Work out the finished part from the listing and answer in its coordinate system (mm). A direction names the side the tool comes from. Give positions to 0.01 mm unless a question says otherwise; leave off trailing zeros. Loops run counter-clockwise (first coordinate to the right, second up) from the corner with the lowest first, then second, coordinate; pieces in that order, holes last.
from build123d import *

# Parameters (mm, degrees)
SKETCH1_W           = 325
SKETCH1_H           = 10
SKETCH1_W_2         = 10
SKETCH1_H_2         = 34.925125471
BOSS_EXTRUDE1_DEPTH = 190
SKETCH2_W           = 190
SKETCH2_H           = 7.5
BOSS_EXTRUDE2_DEPTH = 5
SKETCH6_W           = 43.6
SKETCH6_H           = 10
BOSS_EXTRUDE4_DEPTH = 190
CUT_EXTRUDE1_START  = -45.92512547
SKETCH3_W           = 153.75
SKETCH3_H           = 43.596922071
CUT_EXTRUDE1_DEPTH  = 56.92512547
SKETCH4_R           = 2.5
BOSS_EXTRUDE3_DEPTH = 171.875
LPATTERN1_COUNT     = 2
LPATTERN1_PITCH     = 190
SKETCH7_W           = 176
SKETCH7_H           = 27.925125471
CUT_EXTRUDE5_DEPTH  = 315
SKETCH8_W           = 25
SKETCH8_H           = 10
BOSS_EXTRUDE6_DEPTH = 325


with BuildPart() as part:
    # Sketch1 → Boss-Extrude1 (new body)
    with BuildSketch(Plane(origin=(0, 0, 0), x_dir=(0, 0, -1), z_dir=(1, 0, 0))):
        with Locations((0, -9.857682562)):
            Rectangle(SKETCH1_W, SKETCH1_H)
        with Locations((-157.5, 12.604880173)):
            Rectangle(SKETCH1_W_2, SKETCH1_H_2)
        with Locations((157.5, 12.604880173)):
            Rectangle(SKETCH1_W_2, SKETCH1_H_2)
    extrude(amount=BOSS_EXTRUDE1_DEPTH)

    # Sketch2 → Boss-Extrude2 (add)
    with BuildSketch(Plane.XZ.offset(14.857682562)):
        with Locations((95, 141.030384385)):
            Rectangle(SKETCH2_W, SKETCH2_H)
        with Locations((95, -141.03)):
            Rectangle(SKETCH2_W, SKETCH2_H)
    extrude(amount=BOSS_EXTRUDE2_DEPTH)

    # Sketch6 → Boss-Extrude4 (add, through all)
    with BuildSketch(Plane.ZY):
        with Locations((90.204898917, -19.857682562)):
            Rectangle(SKETCH6_W, SKETCH6_H)
    boss_extrude4 = extrude(amount=-BOSS_EXTRUDE4_DEPTH)

    # Sketch3 → Cut-Extrude1 (cut)
    with BuildSketch(Plane.XZ.offset(14.857682562).offset(CUT_EXTRUDE1_START)):
        with Locations((95, 89.856251598)):
            Rectangle(SKETCH3_W, SKETCH3_H)
    cut_extrude1 = extrude(amount=CUT_EXTRUDE1_DEPTH, mode=Mode.SUBTRACT)

    # Sketch4 → Boss-Extrude3 (add, through all)
    with BuildSketch(Plane.ZY.offset(-171.875)):
        with Locations((90.207259337, -15.987312382)):
            Circle(SKETCH4_R)
    boss_extrude3 = extrude(amount=BOSS_EXTRUDE3_DEPTH)

    # LPattern1: Boss-Extrude4, Cut-Extrude1, Boss-Extrude3 ×2
    with Locations(*[(0, 0, -i * LPATTERN1_PITCH) for i in range(1, LPATTERN1_COUNT)]):
        add(boss_extrude4)
        add(cut_extrude1, mode=Mode.SUBTRACT)
        add(boss_extrude3)

    # Sketch7 → Cut-Extrude5 (cut)
    with BuildSketch(Plane(origin=(0, 0, 152.5), x_dir=(-1, 0, 0), z_dir=(0, 0, -1))):
        with Locations((-95, 9.104880173)):
            Rectangle(SKETCH7_W, SKETCH7_H)
    extrude(amount=CUT_EXTRUDE5_DEPTH, mode=Mode.SUBTRACT)

    # Sketch8 → Boss-Extrude6 (add)
    with BuildSketch(Plane(origin=(0, 0, -162.5), x_dir=(-1, 0, 0), z_dir=(0, 0, -1))):
        with Locations((12.5, -9.857682562)):
            Rectangle(SKETCH8_W, SKETCH8_H)
    extrude(amount=-BOSS_EXTRUDE6_DEPTH)


solid = part.part
Item 1: Find section B-B, the plane y = -9. Write down the section's boundary in (x, z) (3 decimals).
Item 2: Consider line 1 (Z direction, x = 119, y = -11); line 2 (Z direction, x = 128, y = -19); line 3 (Z direction, x = 46.5, y = -22). Determine where each line is inside the solid, lowest interval first.
Item 3: Find section D-D, the plane x = 166. Give the number of separate pieces and of enclosed holes in the cut face, plus the area to 3 significant figures.
Item 4: For faces 4 (the face through (96, 23.067, -157)), 5 (the face through (0, 13, 158)), 6 (the face through (94, -15, 111.655)), 7 (the face through (94, -20, -77.995)), determine the directions among +Z, -Z, +X, -X, +Y, -Y from which every point of the face is accessible in a straight line to the end or side of a thin tool.
Item 5: Determine the mould class of faces 1 (the face through (94, -10, -121.942)), 2 (the face through (0, -20, 91)), 3 (the face through (94, -19.858, -141)) for opening direction X: released by +X, released by -X, zero draft, split by the parting line, or undercut.
Item 6: Find section A-A, the plane y = 12. Write down the section's boundary in (x, z), plus the area to 3 significant figures.
Item 7: Flat-ended cylindrical pins translate along their axes: pin 1 Ø8 at (y, z) = (5, -156.5) entering from -X; pin 2 Ø6 at (x, y) = (72, -16) entering from -Z; pin 3 Ø3 at (x, y) = (9.5, -19.5) entering from -Z; pin 4 Ø2.5 at (x, y) = (106.5, -18) entering from +Z. Find the tip coordinate at first contact, or state that the pin passes through.
Item 8: Find section C-C, the plane z = -81.5. Write down the section's boundary in (x, y) (3 decimals), plus the area to 3 significant figures.
Ans:
1. outline: (-25, -162.5) - (190, -162.5) - (190, 162.5) - (-25, 162.5) - close; hole (18.125, -121.942) - (171.875, -121.942) - (171.875, -78.345) - (18.125, -78.345) - close; hole (18.125, 68.058) - (171.875, 68.058) - (171.875, 111.655) - (18.125, 111.655) - close
2. line 1: z = -162.5 to -121.94, -78.35 to 68.06, 111.65 to 162.5
2. line 2: z = -144.78 to -137.28, -78.35 to -78, 111.65 to 112, 137.28 to 144.78
2. line 3: z = -78.35 to -78, 111.65 to 112
3. separate pieces: 6
3. enclosed holes: 0
3. area: 2,920 mm2
4. face 4: -Z
4. face 5: +Z, -Z, -X, +Y
4. face 6: +Y, -Y
4. face 7: +X, -X, -Y
5. face 1: undercut
5. face 2: released by -X
5. face 3: zero draft
6. outline: (0, -162.5) - (7, -162.5) - (7, -152.5) - (0, -152.5) - close; (0, 152.5) - (190, 152.5) - (190, 162.5) - (0, 162.5) - close; (183, -162.5) - (190, -162.5) - (190, -152.5) - (183, -152.5) - close
6. area: 2,040 mm2
7. pin 1: stops at x = 0
7. pin 2: stops at z = -162.5
7. pin 3: stops at z = -144.78
7. pin 4: stops at z = 144.78
8. outline: (-25, -14.858) - (0, -14.858) - (0, -24.858) - (18.125, -24.858) - (18.125, -4.858) - (-25, -4.858) - close; (171.875, -24.858) - (190, -24.858) - (190, -4.858) - (171.875, -4.858) - close
8. area: 975 mm2
